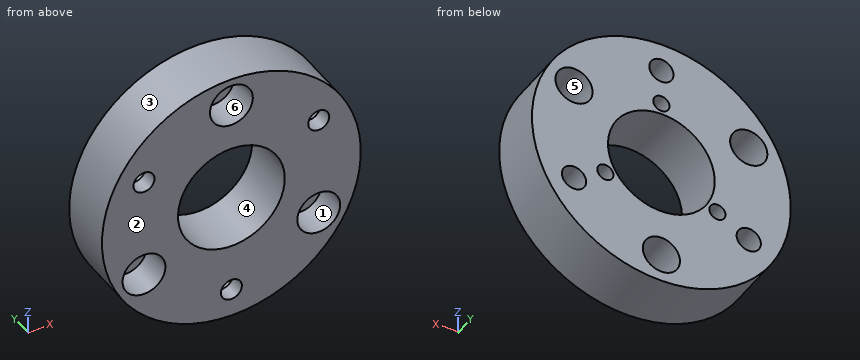
```python
from build123d import *

# Parameters (mm, degrees)
SKETCH_1_R          = 16
SKETCH_1_R_2        = 6.6
SKETCH_1_R_3        = 1.3
EXTRUDE_1_DEPTH     = 7
SKETCH_2_R          = 2.3
CUT_EXTRUDE_2_DEPTH = 5
SKETCH_4_R          = 1
CUT_EXTRUDE_3_DEPTH = 2
SKETCH_5_R          = 1.5
CUT_EXTRUDE_4_DEPTH = 34.400366855
SKETCH_6_R          = 2.65
CUT_EXTRUDE_5_DEPTH = 4


with BuildPart() as part:
    # 草图1 → 凸台-拉伸1 (new body)
    with BuildSketch(Plane(origin=(0, 0, 0), x_dir=(1, 0, 0), z_dir=(0, 1, 0))):
        with Locations(Location((0, -12.470765814, 0), (0, 0, 270))):
            Circle(SKETCH_1_R)
        with Locations(Location((0, -12.470765814, 0), (0, 0, 270))):
            Circle(SKETCH_1_R_2, mode=Mode.SUBTRACT)
        with Locations(Location((-10.8, -18.706148722, 0), (0, 0, 270))):
            Circle(SKETCH_1_R_3, mode=Mode.SUBTRACT)
        with Locations(Location((10.8, -18.706148722, 0), (0, 0, 270))):
            Circle(SKETCH_1_R_3, mode=Mode.SUBTRACT)
        with Locations(Location((0, 0, 0), (0, 0, 270))):
            Circle(SKETCH_1_R_3, mode=Mode.SUBTRACT)
    extrude(amount=EXTRUDE_1_DEPTH)

    # 草图2 → 切除-拉伸2 (cut)
    with BuildSketch(Plane(origin=(0, 7, 0), x_dir=(1, 0, 0), z_dir=(0, 1, 0))):
        with Locations(Location((-10.8, -18.706148722, 0), (0, 0, 270))):
            Circle(SKETCH_2_R)
        with Locations(Location((10.8, -18.706148722, 0), (0, 0, 270))):
            Circle(SKETCH_2_R)
        with Locations(Location((0, 0, 0), (0, 0, 270))):
            Circle(SKETCH_2_R)
    extrude(amount=-CUT_EXTRUDE_2_DEPTH, mode=Mode.SUBTRACT)

    # 草图4 → 切除-拉伸3 (cut)
    with BuildSketch(Plane(origin=(0, 7, 0), x_dir=(1, 0, 0), z_dir=(0, 1, 0))):
        with Locations(Location((-6.92820323, -8.470765814, 0), (0, 0, 270))):
            Circle(SKETCH_4_R)
        with Locations(Location((6.92820323, -8.470765814, 0), (0, 0, 90))):
            Circle(SKETCH_4_R)
        with Locations(Location((0, -20.470765814, 0), (0, 0, 270))):
            Circle(SKETCH_4_R)
    extrude(amount=-CUT_EXTRUDE_3_DEPTH, mode=Mode.SUBTRACT)

    # 草图5 → 切除-拉伸4 (cut, through all)
    with BuildSketch(Plane(origin=(0, 7, 0), x_dir=(1, 0, 0), z_dir=(0, 1, 0))):
        with Locations(Location((-10.8, -6.235382907, 0), (0, 0, 270))):
            Circle(SKETCH_5_R)
        with Locations(Location((10.8, -6.235382907, 0), (0, 0, 270))):
            Circle(SKETCH_5_R)
        with Locations(Location((0, -24.941531629, 0), (0, 0, 270))):
            Circle(SKETCH_5_R)
    extrude(amount=-CUT_EXTRUDE_4_DEPTH, mode=Mode.SUBTRACT)

    # 草图6 → 切除-拉伸5 (cut)
    with BuildSketch(Plane.XZ):
        with Locations(Location((0, 24.941531629, 0), (0, 0, 270))):
            Circle(SKETCH_6_R)
        with Locations(Location((-10.8, 6.235382907, 0), (0, 0, 270))):
            Circle(SKETCH_6_R)
        with Locations(Location((10.8, 6.235382907, 0), (0, 0, 270))):
            Circle(SKETCH_6_R)
    extrude(amount=-CUT_EXTRUDE_5_DEPTH, mode=Mode.SUBTRACT)


solid = part.part
```
The listing builds one solid part. Answer for the finished solid, in the listing's coordinates (mm). Face numbers are marked on the shaded views. A direction names the side the tool comes from. Give positions to 0.01 mm unless a question says otherwise; leave off trailing zeros. Order: outer loops, then holes, each group sorted by start corner. A loop starts at its lowest first (then second) coordinate and runs counter-clockwise, first axis right, second up. Notation, with made-up numbers: M 78,76.25 L 95,76.25 A26 cw 95,96.25 Z; hole C 85,8.5 d7. An arc over 180 degrees is marked long. Put each result on its own line as item: value. Start each with the question number.
Item 1: Find the intervals of material crossed by line 1 along X through (y, z) = (1, 5); line 2 along Z through (x, y) = (12, 3.5); line 3 along X through (y, z) = (6.25, 17), in increasing order.
Item 2: The part is cut by section A-A, the plane y = 3. Determine the outline of the cut face in (x, z).
Item 3: The part is cut by section B-B, the plane x = 0. Determine the outline of the cut face in (y, z).
Item 4: Flat-ended cylindrical pins translate along their axes: P1, Ø4, axis at x = 0, z = 0, coming from the +Y side; P2, Ø1, axis at x = -10, y = 0.5, coming from the +Z side; P3, Ø5, axis at x = -10.8, z = 6.24, coming from the -Y side. Find the tip coordinate at first contact, or state that the pin passes through.
Item 5: For a pull along X with two mould halves and no side action, classify the marked faces 1, 2 and 3 as +X half, -X half, draft (parallel to the pull), parting line (faces both ways), or undercut.
Item 6: The part is cut by section D-D, the plane x = -10.8. Determine the outline of the cut face in (y, z).
Item 7: The part is cut by section C-C, the plane z = 18.5. Determine the outline of the cut face in (x, y), and give its area (3 significant figures).
Item 8: Which of the six approach directions +Z, -Z, +X, -X, +Y, -Y give full straight-line access (tool end or side, diameter ignored) to the marked faces 4, 5 and 6?
Answer key:
1. line 1: x = -14.15 to -13.14, -8.46 to 8.46, 13.14 to 14.15
1. line 2: z = 1.89 to 3.87, 8.6 to 16.74, 20.67 to 23.05
1. line 3: x = -15.35 to -12.34, -9.26 to -4.8, 4.8 to 9.26, 12.34 to 15.35
2. outline: C 0,12.47 d32; hole C -10.8,6.24 d5.3; hole C -10.8,18.71 d4.6; hole C 0,12.47 d13.2; hole C 0,24.94 d5.3; hole C 0,0 d4.6; hole C 10.8,6.24 d5.3; hole C 10.8,18.71 d4.6
3. outline: M 0,-3.53 L 7,-3.53 L 7,-2.3 L 2,-2.3 L 2,-1.3 L 0,-1.3 Z; M 0,1.3 L 2,1.3 L 2,2.3 L 7,2.3 L 7,5.87 L 0,5.87 Z; M 0,19.07 L 7,19.07 L 7,19.47 L 5,19.47 L 5,21.47 L 7,21.47 L 7,23.44 L 4,23.44 L 4,22.29 L 0,22.29 Z; M 0,27.59 L 4,27.59 L 4,26.44 L 7,26.44 L 7,28.47 L 0,28.47 Z
4. P1: stops at y = 2
4. P2: stops at z = 25.35
4. P3: stops at y = 4
5. face 1: undercut
5. face 2: draft
5. face 3: parting line
6. outline: M 0,0.67 L 7,0.67 L 7,4.74 L 4,4.74 L 4,3.59 L 0,3.59 Z; M 0,8.89 L 4,8.89 L 4,7.74 L 7,7.74 L 7,16.41 L 2,16.41 L 2,17.41 L 0,17.41 Z; M 0,20.01 L 2,20.01 L 2,21.01 L 7,21.01 L 7,24.28 L 0,24.28 Z
7. outline: M -14.82,0 L -12.08,0 L -12.08,2 L -13.09,2 L -13.09,7 L -14.82,7 Z; M -9.52,0 L -2.68,0 L -2.68,7 L -8.51,7 L -8.51,2 L -9.52,2 Z; M 2.68,0 L 9.52,0 L 9.52,2 L 8.51,2 L 8.51,7 L 2.68,7 Z; M 12.08,0 L 14.82,0 L 14.82,7 L 13.09,7 L 13.09,2 L 12.08,2 Z
7. area: 114 mm²
8. face 4: +Y, -Y
8. face 5: +Y
8. face 6: -Y
